```python
from build123d import *

# Parameters (mm, degrees)
EXTRUDE1_DEPTH          = 1
FILLET1_R               = 1.2
CUT_EXTRUDE1_DEPTH      = 12.181737343
CUT_EXTRUDE1_DEPTH_BACK = 12.181737343
CHAMFER1_SIZE           = 0.25


with BuildPart() as part:
    # Sketch1 → Extrude1 (new, symmetric)
    with BuildSketch(Plane(origin=(0, 0, 0), x_dir=(0, 0, -1), z_dir=(1, 0, 0))):
        with BuildLine():
            Line((-6.381117354, -4.614863629), (-2.317843826, -3.26))
            ThreePointArc((-2.317843826, -3.26), (-1.216552506, -3.810511777), (0, -4))
            Line((0, -4), (0, -6.129032258))
            ThreePointArc((0, -6.129032258), (3.615250795, -4.949242175), (5.8386874, -1.864072388))
            Line((5.8386874, -1.864072388), (3.810511777, -1.216552506))
            ThreePointArc((3.810511777, -1.216552506), (4, 0), (3.810511777, 1.216552506))
            Line((3.810511777, 1.216552506), (5.8386874, 1.864072388))
            ThreePointArc((5.8386874, 1.864072388), (3.615250795, 4.949242175), (0, 6.129032258))
            Line((0, 6.129032258), (0, 4))
            ThreePointArc((0, 4), (-1.216552506, 3.810511777), (-2.317843826, 3.26))
            Line((-2.317843826, 3.26), (-6.381117354, 4.614863629))
            ThreePointArc((-6.381117354, 4.614863629), (7.875, 0), (-6.381117354, -4.614863629))
        make_face()
    extrude(amount=EXTRUDE1_DEPTH, both=True)

    # Fillet1
    fillet1_edges = [part.edges().sort_by_distance(p)[0] for p in [
        (0, -4.614863629, 6.381117354),
        (0, -6.129032258, 0),
        (0, -1.864072388, -5.8386874),
        (0, 1.864072388, -5.8386874),
        (0, 6.129032258, 0),
        (0, 4.614863629, 6.381117354),
    ]]
    fillet(fillet1_edges, radius=FILLET1_R)

    # Sketch4 → Cut-Extrude1 (cut, two sides: drawn at the far end of the back side and taken through both)
    with BuildSketch(Plane(origin=(0, 0, 0), x_dir=(0, 0, -1), z_dir=(1, 0, 0)).offset(-CUT_EXTRUDE1_DEPTH_BACK)):
        with BuildLine():
            Line((0, 4.780727874), (0, -4.780727874))
            ThreePointArc((0, -4.780727874), (0.461953903, -5.726924448), (1.492146597, -5.944622356))
            ThreePointArc((1.492146597, -5.944622356), (3.615250795, -4.949242175), (5.209194703, -3.229446851))
            ThreePointArc((5.209194703, -3.229446851), (5.315130469, -2.181846269), (4.554254966, -1.454001619))
            ThreePointArc((4.554254966, -1.454001619), (4, 0), (4.554254966, 1.454001619))
            ThreePointArc((4.554254966, 1.454001619), (5.315130469, 2.181846269), (5.209194703, 3.229446851))
            ThreePointArc((5.209194703, 3.229446851), (3.615250795, 4.949242175), (1.492146597, 5.944622356))
            ThreePointArc((1.492146597, 5.944622356), (0.461953903, 5.726924448), (0, 4.780727874))
        make_face()
    extrude(amount=CUT_EXTRUDE1_DEPTH + CUT_EXTRUDE1_DEPTH_BACK, mode=Mode.SUBTRACT)

    # Chamfer1
    # the kernel refuses this chamfer: 0.25 mm, written as the material it takes off along each edge
    with BuildSketch(Plane(origin=(1, 3.056631288, 1.707935428), x_dir=(0, 0.9486525372163972, -0.31632003356235944), z_dir=(0, 0.31632003356235944, 0.9486525372163972)), Plane(origin=(-1, 3.056631288, 1.707935428), x_dir=(1, 0, 0), z_dir=(0, 0.31632003356235944, 0.9486525372163972)), Plane(origin=(-1, -4.370192178, 5.647340899), x_dir=(1, 0, 0), z_dir=(0, 0.3163200335623596, -0.9486525372163971))) as chamfer1_piece_1:
        Polygon((CHAMFER1_SIZE, 0), (0, CHAMFER1_SIZE), (0, 0), align=None)
    extrude(amount=4.15263262, mode=Mode.SUBTRACT)
    with BuildSketch(Plane(origin=(1, 0, 0), x_dir=(0, 0.9871090886928867, -0.16004888946787105), z_dir=(0, -0.16004888946787105, -0.9871090886928867))) as chamfer1_piece_2:
        Polygon((4 + CHAMFER1_SIZE, 0), (4, -CHAMFER1_SIZE), (4, 0), align=None)
    revolve(axis=Axis((1, 0, 0), (1, 0, 0)), revolution_arc=53.832106013, mode=Mode.SUBTRACT)
    with BuildSketch(Plane(origin=(1, 4.780727874, -1.2), x_dir=(0, 0, 1), z_dir=(0, -1, 0))) as chamfer1_piece_3:
        Polygon((1.2 + CHAMFER1_SIZE, 0), (1.2, CHAMFER1_SIZE), (1.2, 0), align=None)
    revolve(axis=Axis((1, 4.780727874, -1.2), (-1, 0, 0)), revolution_arc=104.090576784, mode=Mode.SUBTRACT)
    with BuildSketch(Plane(origin=(1, 0, 0), x_dir=(0, 0.5269097493911834, -0.8499212410550288), z_dir=(0, -0.8499212410550288, -0.5269097493911834))) as chamfer1_piece_4:
        Polygon((6.129032258 + CHAMFER1_SIZE, 0), (6.129032258, -CHAMFER1_SIZE), (6.129032258, 0), align=None)
    revolve(axis=Axis((1, 0, 0), (1, 0, 0)), revolution_arc=44.112527376, mode=Mode.SUBTRACT)
    with BuildSketch(Plane(origin=(1, 2.597155152, -4.189289214), x_dir=(0, 0.5269097493911832, -0.8499212410550289), z_dir=(0, 0.8499212410550289, 0.5269097493911832))) as chamfer1_piece_5:
        Polygon((1.2 + CHAMFER1_SIZE, 0), (1.2, CHAMFER1_SIZE), (1.2, 0), align=None)
    revolve(axis=Axis((1, 2.597155152, -4.189289214), (-1, 0, 0)), revolution_arc=134.804277629, mode=Mode.SUBTRACT)
    with BuildSketch(Plane(origin=(1, 0, -6.18430093), x_dir=(0, 0.8535787339825979, 0.5209638614075505), z_dir=(0, 0.5209638614075505, -0.8535787339825979))) as chamfer1_piece_6:
        Polygon((2.18430093 - CHAMFER1_SIZE, 0), (2.18430093, -CHAMFER1_SIZE), (2.18430093, 0), align=None)
    revolve(axis=Axis((1, 0, -6.18430093), (1, 0, 0)), revolution_arc=117.206144707, mode=Mode.SUBTRACT)
    with BuildSketch(Plane(origin=(1, -2.597155152, -4.189289214), x_dir=(0, 0.9743410747854011, 0.22507658693437918), z_dir=(0, -0.22507658693437918, 0.9743410747854011))) as chamfer1_piece_7:
        Polygon((1.2 + CHAMFER1_SIZE, 0), (1.2, CHAMFER1_SIZE), (1.2, 0), align=None)
    revolve(axis=Axis((1, -2.597155152, -4.189289214), (-1, 0, 0)), revolution_arc=134.804277629, mode=Mode.SUBTRACT)
    with BuildSketch(Plane(origin=(1, 0, 0), x_dir=(0, -0.9699120685888933, -0.24345549738219877), z_dir=(0, -0.24345549738219877, 0.9699120685888933))) as chamfer1_piece_8:
        Polygon((6.129032258 + CHAMFER1_SIZE, 0), (6.129032258, -CHAMFER1_SIZE), (6.129032258, 0), align=None)
    revolve(axis=Axis((1, 0, 0), (1, 0, 0)), revolution_arc=44.112527376, mode=Mode.SUBTRACT)
    with BuildSketch(Plane(origin=(1, -4.780727874, -1.2), x_dir=(0, -0.9699120685888935, -0.24345549738219882), z_dir=(0, 0.24345549738219882, -0.9699120685888935))) as chamfer1_piece_9:
        Polygon((1.2 + CHAMFER1_SIZE, 0), (1.2, CHAMFER1_SIZE), (1.2, 0), align=None)
    revolve(axis=Axis((1, -4.780727874, -1.2), (-1, 0, 0)), revolution_arc=104.090576784, mode=Mode.SUBTRACT)
    with BuildSketch(Plane(origin=(1, -3.357079253, 0), x_dir=(0, 0, 1), z_dir=(0, -1, 0)), Plane(origin=(-1, 4.780727874, 0), x_dir=(1, 0, 0), z_dir=(0, -1, 0)), Plane(origin=(-1, -3.357079253, 0), x_dir=(1, 0, 0), z_dir=(0, -1, 0)), Plane(origin=(1, 4.780727874, 0), x_dir=(0, 0, 1), z_dir=(0, -1, 0))) as chamfer1_piece_10:
        Polygon((CHAMFER1_SIZE, 0), (0, CHAMFER1_SIZE), (0, 0), align=None)
    extrude(amount=1.423648621, mode=Mode.SUBTRACT)
    with BuildSketch(Plane(origin=(1, 0, 0), x_dir=(0, -0.7117518247217879, 0.702431021528239), z_dir=(0, 0.702431021528239, 0.7117518247217879))) as chamfer1_piece_11:
        Polygon((4 + CHAMFER1_SIZE, 0), (4, -CHAMFER1_SIZE), (4, 0), align=None)
    revolve(axis=Axis((1, 0, 0), (1, 0, 0)), revolution_arc=53.832106013, mode=Mode.SUBTRACT)
    with BuildSketch(Plane(origin=(1, -4.370192178, 5.647340899), x_dir=(-1, 0, 0), z_dir=(0, 0.3163200335623596, -0.9486525372163971))) as chamfer1_piece_12:
        Polygon((CHAMFER1_SIZE, 0), (0, -CHAMFER1_SIZE), (0, 0), align=None)
    extrude(amount=4.15263262, mode=Mode.SUBTRACT)
    with BuildSketch(Plane(origin=(-1, 0, 0), x_dir=(0, 0.9871090886928867, -0.16004888946787105), z_dir=(0, -0.16004888946787105, -0.9871090886928867))) as chamfer1_piece_13:
        Polygon((4, CHAMFER1_SIZE), (4 + CHAMFER1_SIZE, 0), (4, 0), align=None)
    revolve(axis=Axis((-1, 0, 0), (1, 0, 0)), revolution_arc=53.832106013, mode=Mode.SUBTRACT)
    with BuildSketch(Plane(origin=(-1, 4.780727874, -1.2), x_dir=(0, 0, 1), z_dir=(0, -1, 0))) as chamfer1_piece_14:
        Polygon((1.2, -CHAMFER1_SIZE), (1.2 + CHAMFER1_SIZE, 0), (1.2, 0), align=None)
    revolve(axis=Axis((-1, 4.780727874, -1.2), (-1, 0, 0)), revolution_arc=104.090576784, mode=Mode.SUBTRACT)
    with BuildSketch(Plane(origin=(-1, 0, 0), x_dir=(0, 0.5269097493911834, -0.8499212410550288), z_dir=(0, -0.8499212410550288, -0.5269097493911834))) as chamfer1_piece_15:
        Polygon((6.129032258, CHAMFER1_SIZE), (6.129032258 + CHAMFER1_SIZE, 0), (6.129032258, 0), align=None)
    revolve(axis=Axis((-1, 0, 0), (1, 0, 0)), revolution_arc=44.112527376, mode=Mode.SUBTRACT)
    with BuildSketch(Plane(origin=(-1, 2.597155152, -4.189289214), x_dir=(0, 0.5269097493911832, -0.8499212410550289), z_dir=(0, 0.8499212410550289, 0.5269097493911832))) as chamfer1_piece_16:
        Polygon((1.2, -CHAMFER1_SIZE), (1.2 + CHAMFER1_SIZE, 0), (1.2, 0), align=None)
    revolve(axis=Axis((-1, 2.597155152, -4.189289214), (-1, 0, 0)), revolution_arc=134.804277629, mode=Mode.SUBTRACT)
    with BuildSketch(Plane(origin=(-1, 0, -6.18430093), x_dir=(0, -0.8535787339825973, 0.5209638614075514), z_dir=(0, -0.5209638614075514, -0.8535787339825973))) as chamfer1_piece_17:
        Polygon((2.18430093, -CHAMFER1_SIZE), (2.18430093 - CHAMFER1_SIZE, 0), (2.18430093, 0), align=None)
    revolve(axis=Axis((-1, 0, -6.18430093), (-1, 0, 0)), revolution_arc=117.206144707, mode=Mode.SUBTRACT)
    with BuildSketch(Plane(origin=(-1, -2.597155152, -4.189289214), x_dir=(0, 0.9743410747854011, 0.22507658693437918), z_dir=(0, -0.22507658693437918, 0.9743410747854011))) as chamfer1_piece_18:
        Polygon((1.2, -CHAMFER1_SIZE), (1.2 + CHAMFER1_SIZE, 0), (1.2, 0), align=None)
    revolve(axis=Axis((-1, -2.597155152, -4.189289214), (-1, 0, 0)), revolution_arc=134.804277629, mode=Mode.SUBTRACT)
    with BuildSketch(Plane(origin=(-1, 0, 0), x_dir=(0, -0.9699120685888933, -0.24345549738219877), z_dir=(0, -0.24345549738219877, 0.9699120685888933))) as chamfer1_piece_19:
        Polygon((6.129032258, CHAMFER1_SIZE), (6.129032258 + CHAMFER1_SIZE, 0), (6.129032258, 0), align=None)
    revolve(axis=Axis((-1, 0, 0), (1, 0, 0)), revolution_arc=44.112527376, mode=Mode.SUBTRACT)
    with BuildSketch(Plane(origin=(-1, -4.780727874, -1.2), x_dir=(0, -0.9699120685888935, -0.24345549738219882), z_dir=(0, 0.24345549738219882, -0.9699120685888935))) as chamfer1_piece_20:
        Polygon((1.2, -CHAMFER1_SIZE), (1.2 + CHAMFER1_SIZE, 0), (1.2, 0), align=None)
    revolve(axis=Axis((-1, -4.780727874, -1.2), (-1, 0, 0)), revolution_arc=104.090576784, mode=Mode.SUBTRACT)
    with BuildSketch(Plane(origin=(-1, 0, 0), x_dir=(0, -0.7117518247217879, 0.702431021528239), z_dir=(0, 0.702431021528239, 0.7117518247217879))) as chamfer1_piece_21:
        Polygon((4, CHAMFER1_SIZE), (4 + CHAMFER1_SIZE, 0), (4, 0), align=None)
    revolve(axis=Axis((-1, 0, 0), (1, 0, 0)), revolution_arc=53.832106013, mode=Mode.SUBTRACT)


solid = part.part
```
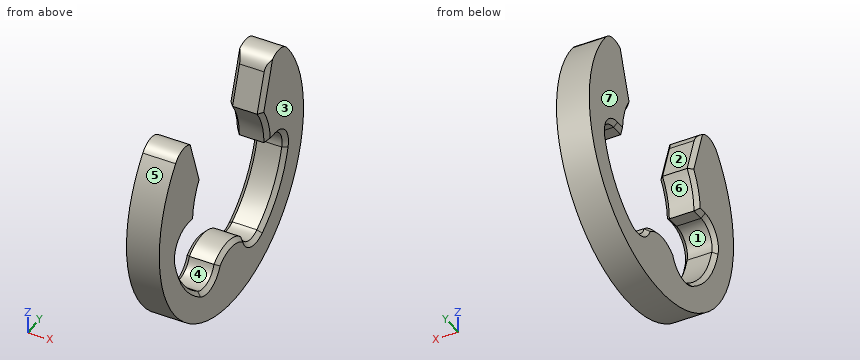
CAD build for the part. Positions are in the model's coordinates, mm. Face numbers are marked on the shaded views. A direction names the side the tool comes from. Round coordinates to 2 decimals unless told otherwise and drop trailing zeros. Loops run counter-clockwise (first coordinate to the right, second up) from the corner with the lowest first, then second, coordinate; pieces in that order, holes last. Notation, with made-up numbers: M 48.25,58.5 L 64.25,58.5 A20 ccw 64.25,68.5 Z; hole C 28,84 d11. An arc over 180 degrees is marked long. Return JSON: item names as keys, results as strings. Group by question number.
(1) Saw through at D-D, the plane y = -6.5. List the corners of the cut face in (x, z), and give its area (3 significant figures).
(2) Drop a flat-ended pin along its axis: P1, Ø0.9, axis at x = 0.5, y = -4.5, coming from the -Z side. Give the stop position or say it passes through.
(3) Mould opens along Z. For the marked faces 4, 5, 6 and 7 say: +Z half, -Z half, draft (parallel to the pull), parting line (faces both ways), or undercut.
(4) Wall check: probe 1 along Y at (x, z) = (-0.65, -5.25); probe 2 along Y at (x, z) = (0, 4.5); probe 3 along Y at (x, z) = (-0.45, 2). Give the ranges that are in metal, low to high. Write a range as [from, to].
(5) Saw through at C-C, the plane z = -4.25. Give the number of separate pieces and of enclosed holes in the cut face, and give its area (3 significant figures).
(6) Tool access for the marked faces 1, 2 and 3: list every direction of +Z, -Z, +X, -X, +Y, -Y with a clear straight run to the whole face (end or side of a thin tool).
(7) Saw through at A-A, the plane y = 0. List the corners of the cut face in (x, z) (3 decimals).
Answer list:
{
 "1": {"outline": "M -1,-4.45 L 1,-4.45 L 1,4.45 L -1,4.45 Z", "area": "17.8 mm2"},
 "2": {"P1": "z = -6.75"},
 "3": {"face 4": "+Z half", "face 5": "parting line", "face 6": "undercut", "face 7": "draft"},
 "4": {"probe 1": "[-5.87, -3.16], [-2.04, 2.04], [3.16, 5.87]", "probe 2": "[-6.46, -3.99], [3.99, 6.46]", "probe 3": "[-7.62, -3.46], [3.46, 7.62]"},
 "5": {"separate pieces": "3", "enclosed holes": "0", "area": "12.4 mm2"},
 "6": {"face 1": "+X, -X", "face 2": "+Z, +X, -X", "face 3": "+Z, -Z, +X, +Y, -Y"},
 "7": {"outline": "M -1,-7.875 L 1,-7.875 L 1,-4.25 L 0.75,-4 L -0.75,-4 L -1,-4.25 Z"}
}
